Can you work these out from the drawing? Everything is in mm from the part's minimum corner. A direction names the side the tool comes from. Coordinates: 2 decimals unless noted, no trailing zeros. Loops run counter-clockwise (first coordinate to the right, second up) from the corner with the lowest first, then second, coordinate; pieces in that order, holes last. Notation, with made-up numbers: (57.5, 2) -> (77.5, 2) arc R26 cw to (77.5, 37) -> close; hole circle Ø7 at (-39, 71.5). An arc over 180 degrees is marked (long way). Put each result on its own line as item: value. Start each with the question number.
Item 1: For the marked faces 1 and 2, which set-ups out of +Z, -Z, +X, -X, +Y, -Y let a thin tool reach every point of the face, with its end or its side?
Item 2: If we section it at C-C on y = 4.75: Please give me the cut outline in (x, z).
Item 3: Will these pins go through, and if not, where does the flat tip stop? P1, Ø1, axis at x = 4.5, y = 7, coming from the +Z side; P2, Ø1.5, axis at y = 7, z = 3, coming from the -X side; P3, Ø2, axis at x = 3.5, z = 1, coming from the +Y side (1 decimal).
Item 4: Please list where these lines run through material, in increasing order: L1, parallel to Y at x = 5, z = 1.95; L2, parallel to Y at x = 5, z = 0.3; L3, parallel to Z at x = 7.25, y = 4. Write a range as from..to.
Item 5: If we section it at D-D on y = 7: Please give me the cut outline in (x, z).
Item 6: If we section it at A-A on x = 5: Please give me the cut outline in (y, z), plus the area to 3 significant figures.
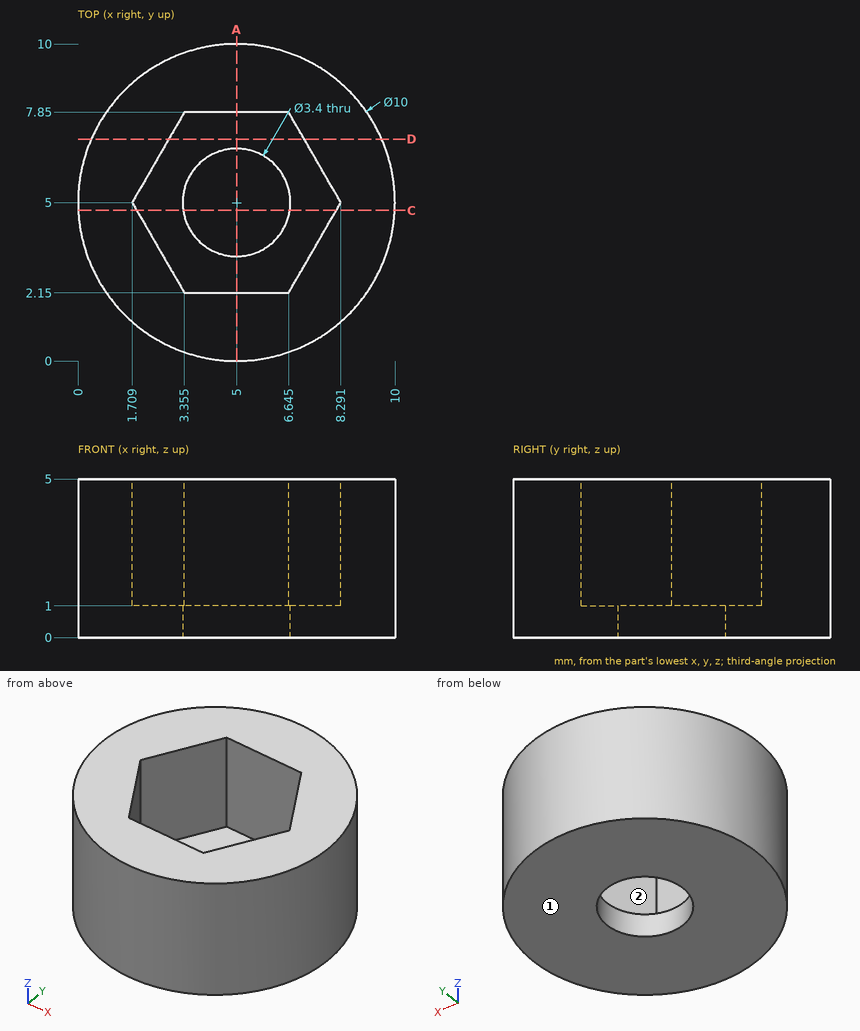
Solutions:
1. face 1: -Z, +X, -X, +Y, -Y
1. face 2: +Z
2. outline: (0.01, 0) -> (3.32, 0) -> (3.32, 1) -> (1.85, 1) -> (1.85, 5) -> (0.01, 5) -> close; (6.68, 0) -> (9.99, 0) -> (9.99, 5) -> (8.15, 5) -> (8.15, 1) -> (6.68, 1) -> close
3. P1: z = 1
3. P2: x = 0.16
3. P3: y = 10
4. L1: 0..2.15, 7.85..10
4. L2: 0..3.3, 6.7..10
4. L3: 0..1
5. outline: (0.42, 0) -> (9.58, 0) -> (9.58, 5) -> (7.14, 5) -> (7.14, 1) -> (2.86, 1) -> (2.86, 5) -> (0.42, 5) -> close
6. outline: (0, 0) -> (3.3, 0) -> (3.3, 1) -> (2.15, 1) -> (2.15, 5) -> (0, 5) -> close; (6.7, 0) -> (10, 0) -> (10, 5) -> (7.85, 5) -> (7.85, 1) -> (6.7, 1) -> close
6. area: 23.8 mm^2
